Design review of the part built by this model. Coordinates are the model's own, in mm. Coordinates: 2 decimals unless noted, no trailing zeros. Loops run counter-clockwise (first coordinate to the right, second up) from the corner with the lowest first, then second, coordinate; pieces in that order, holes last. Notation, with made-up numbers: (50, -10) - (95, -10) arc R24 ccw to (95, 4) - close; hole circle Ø4 at (13, 58). An arc over 180 degrees is marked (long way). Return JSON: item names as keys, results as strings. Group by question number.
from build123d import *

# Parameters (mm, degrees)
SKETCH1_R           = 1.5
SKETCH1_R_2         = 2.286
SKETCH1_R_3         = 2.794
BOSS_EXTRUDE1_DEPTH = 6.35


with BuildPart() as part:
    # Sketch1 → Boss-Extrude1 (new body)
    with BuildSketch(Plane.XY):
        with BuildLine():
            Line((-491.330243723, 4.906575793), (-491.330243723, -1.443424207))
            Line((-491.330243723, -1.443424207), (-491.330243723, -103.680930126))
            ThreePointArc((-491.330243723, -103.680930126), (-482.543447159, -124.894133561), (-461.330243723, -133.680930126))
            Line((-461.330243723, -133.680930126), (-13.330243723, -133.680930126))
            ThreePointArc((-13.330243723, -133.680930126), (7.882959712, -124.894133561), (16.669756277, -103.680930126))
            Line((16.669756277, -103.680930126), (16.669756277, -1.443424207))
            Line((16.669756277, -1.443424207), (16.669756277, 4.906575793))
            Line((16.669756277, 4.906575793), (-8.730243723, 4.906575793))
            Line((-8.730243723, 4.906575793), (-8.730243723, -1.443424207))
            Line((-8.730243723, -1.443424207), (-59.530243723, -1.443424207))
            Line((-59.530243723, -1.443424207), (-59.530243723, 4.906575793))
            Line((-59.530243723, 4.906575793), (-84.930243723, 4.906575793))
            Line((-84.930243723, 4.906575793), (-84.930243723, -1.443424207))
            Line((-84.930243723, -1.443424207), (-135.730243723, -1.443424207))
            Line((-135.730243723, -1.443424207), (-135.730243723, 4.906575793))
            Line((-135.730243723, 4.906575793), (-161.130243723, 4.906575793))
            Line((-161.130243723, 4.906575793), (-161.130243723, -1.443424207))
            Line((-161.130243723, -1.443424207), (-313.530243723, -1.443424207))
            Line((-313.530243723, -1.443424207), (-313.530243723, 4.906575793))
            Line((-313.530243723, 4.906575793), (-338.930243723, 4.906575793))
            Line((-338.930243723, 4.906575793), (-338.930243723, -1.443424207))
            Line((-338.930243723, -1.443424207), (-389.730243723, -1.443424207))
            Line((-389.730243723, -1.443424207), (-389.730243723, 4.906575793))
            Line((-389.730243723, 4.906575793), (-415.130243723, 4.906575793))
            Line((-415.130243723, 4.906575793), (-415.130243723, -1.443424207))
            Line((-415.130243723, -1.443424207), (-465.930243723, -1.443424207))
            Line((-465.930243723, -1.443424207), (-465.930243723, 4.906575793))
            Line((-465.930243723, 4.906575793), (-491.330243723, 4.906575793))
        make_face()
        with Locations((-482.62608839, -103.680930126)):
            Circle(SKETCH1_R, mode=Mode.SUBTRACT)
        with Locations((-357.330243723, -126.721486066)):
            Circle(SKETCH1_R, mode=Mode.SUBTRACT)
        with Locations((-461.780243723, -77.562177166)):
            Circle(SKETCH1_R_2, mode=Mode.SUBTRACT)
        with Locations((-372.880243723, -77.562177166)):
            Circle(SKETCH1_R_2, mode=Mode.SUBTRACT)
        with Locations((-341.780243723, -77.562177166)):
            Circle(SKETCH1_R_2, mode=Mode.SUBTRACT)
        with Locations((-252.880243723, -77.562177166)):
            Circle(SKETCH1_R_2, mode=Mode.SUBTRACT)
        with Locations((-237.330243723, -126.721486066)):
            Circle(SKETCH1_R, mode=Mode.SUBTRACT)
        with Locations((-117.330243723, -126.721486066)):
            Circle(SKETCH1_R, mode=Mode.SUBTRACT)
        with Locations((7.965600943, -103.680930126)):
            Circle(SKETCH1_R, mode=Mode.SUBTRACT)
        with Locations((-221.780243723, -77.562177166)):
            Circle(SKETCH1_R_2, mode=Mode.SUBTRACT)
        with Locations((-132.880243723, -77.562177166)):
            Circle(SKETCH1_R_2, mode=Mode.SUBTRACT)
        with Locations((-101.780243723, -77.562177166)):
            Circle(SKETCH1_R_2, mode=Mode.SUBTRACT)
        with Locations((-12.880243723, -77.562177166)):
            Circle(SKETCH1_R_2, mode=Mode.SUBTRACT)
        with BuildLine():
            ThreePointArc((-482.62608839, -39.813208936), (-477.330243723, -34.51736427), (-472.034399057, -39.813208936))
            Line((-472.034399057, -39.813208936), (-472.034399057, -63.648583111))
            ThreePointArc((-472.034399057, -63.648583111), (-477.330243723, -68.944427778), (-482.62608839, -63.648583111))
            Line((-482.62608839, -63.648583111), (-482.62608839, -39.813208936))
        make_face(mode=Mode.SUBTRACT)
        with BuildLine():
            ThreePointArc((-362.62608839, -39.813208936), (-357.330243723, -34.51736427), (-352.034399057, -39.813208936))
            Line((-352.034399057, -39.813208936), (-352.034399057, -63.648583111))
            ThreePointArc((-352.034399057, -63.648583111), (-357.330243723, -68.944427778), (-362.62608839, -63.648583111))
            Line((-362.62608839, -63.648583111), (-362.62608839, -39.813208936))
        make_face(mode=Mode.SUBTRACT)
        with Locations((-477.330243723, -17.953424207)):
            Circle(SKETCH1_R_3, mode=Mode.SUBTRACT)
        with Locations((-357.330243723, -17.953424207)):
            Circle(SKETCH1_R_3, mode=Mode.SUBTRACT)
        with Locations((-296.221681692, -15.413424207)):
            Circle(SKETCH1_R, mode=Mode.SUBTRACT)
        with BuildLine():
            ThreePointArc((-242.62608839, -39.813208936), (-237.330243723, -34.51736427), (-232.034399057, -39.813208936))
            Line((-232.034399057, -39.813208936), (-232.034399057, -63.648583111))
            ThreePointArc((-232.034399057, -63.648583111), (-237.330243723, -68.944427778), (-242.62608839, -63.648583111))
            Line((-242.62608839, -63.648583111), (-242.62608839, -39.813208936))
        make_face(mode=Mode.SUBTRACT)
        with BuildLine():
            ThreePointArc((-122.62608839, -39.813208936), (-117.330243723, -34.51736427), (-112.034399057, -39.813208936))
            Line((-112.034399057, -39.813208936), (-112.034399057, -63.648583111))
            ThreePointArc((-112.034399057, -63.648583111), (-117.330243723, -68.944427778), (-122.62608839, -63.648583111))
            Line((-122.62608839, -63.648583111), (-122.62608839, -39.813208936))
        make_face(mode=Mode.SUBTRACT)
        with BuildLine():
            ThreePointArc((-2.62608839, -39.813208936), (2.669756277, -34.51736427), (7.965600943, -39.813208936))
            Line((7.965600943, -39.813208936), (7.965600943, -63.648583111))
            ThreePointArc((7.965600943, -63.648583111), (2.669756277, -68.944427778), (-2.62608839, -63.648583111))
            Line((-2.62608839, -63.648583111), (-2.62608839, -39.813208936))
        make_face(mode=Mode.SUBTRACT)
        with Locations((-177.33024378, -15.413424207)):
            Circle(SKETCH1_R, mode=Mode.SUBTRACT)
        with Locations((-117.330243723, -17.953424207)):
            Circle(SKETCH1_R_3, mode=Mode.SUBTRACT)
        with Locations((2.669756277, -17.953424207)):
            Circle(SKETCH1_R_3, mode=Mode.SUBTRACT)
    extrude(amount=BOSS_EXTRUDE1_DEPTH)


solid = part.part
Item 1: To check wall thickness, follow line 1 (X direction, y = -15, z = 3.25); line 2 (X direction, y = -64.5, z = 1); line 3 (X direction, y = -59.5, z = 2.25). State the ranges of each line that lie inside material, in increasing order. Write a range as from..to.
Item 2: Add section A-A (x = -203). State the section outline as (y, z) points, then the cut area to 3 significant figures.
Item 3: Add section B-B (z = 5). Give the number of separate pieces and of enclosed holes in the cut face, then the cut area to 3 significant figures.
Item 4: For P1, Ø6, axis at x = -394, y = -28, coming from the -Z side; P2, Ø1.9, axis at x = -355.5, z = 2.5, coming from the +Y side, all flat-tipped, find the tip position at first contact; note any pin that passes through.
Answers below:
{
 "1": {"line 1": "x = -491.33..-297.66, -294.78..-178.77, -175.89..16.67", "line 2": "x = -491.33..-482.56, -472.1..-362.56, -352.1..-242.56, -232.1..-122.56, -112.1..-2.56, 7.9..16.67", "line 3": "x = -491.33..-482.63, -472.03..-362.63, -352.03..-242.63, -232.03..-122.63, -112.03..-2.63, 7.97..16.67"},
 "2": {"outline": "(-133.68, 0) - (-1.44, 0) - (-1.44, 6.35) - (-133.68, 6.35) - close", "area": "840 mm^2"},
 "3": {"separate pieces": "1", "enclosed holes": "24", "area": "65,800 mm^2"},
 "4": {"P1": "stops at z = 0", "P2": "stops at y = -1.44"}
}
